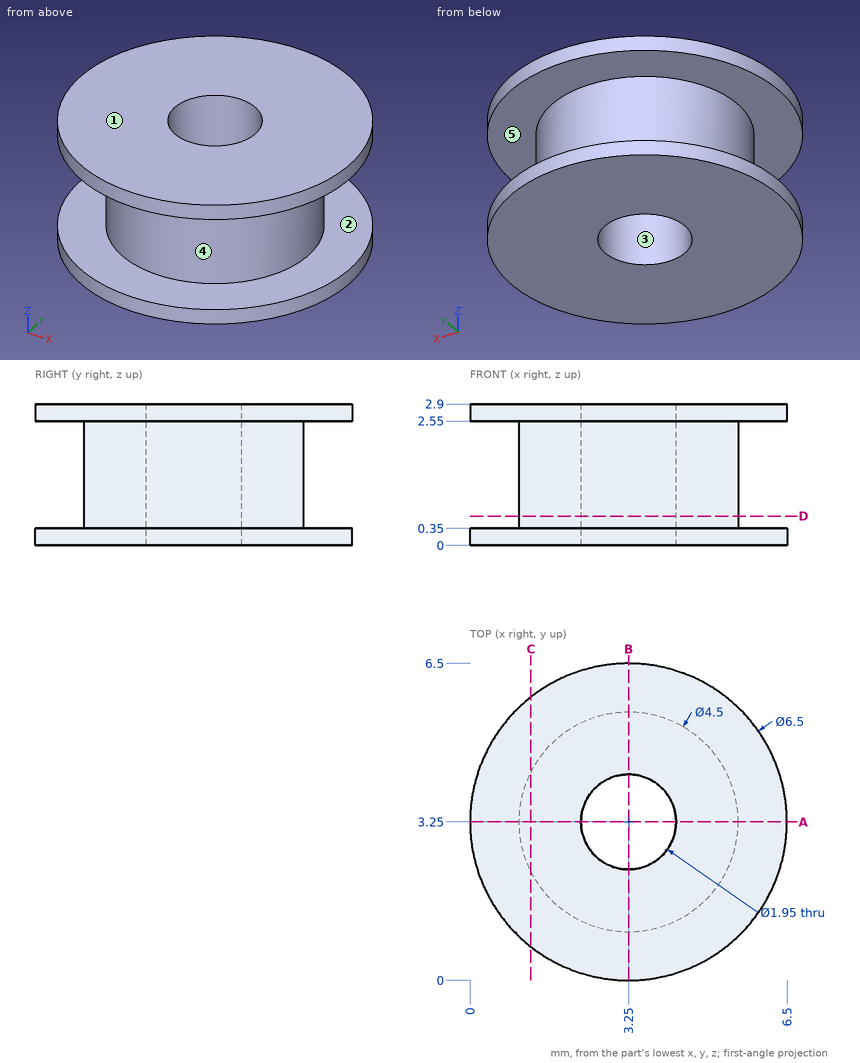
Design review of the part shown in the three views and the two pictorial views. Dimensions are in mm from the part's minimum x, y and z. A direction names the side the tool comes from. Give positions to 0.01 mm unless a question says otherwise; leave off trailing zeros. Loops run counter-clockwise (first coordinate to the right, second up) from the corner with the lowest first, then second, coordinate; pieces in that order, holes last. Notation, with made-up numbers: (64.5, 44.5) -> (77.5, 44.5) arc R19 ccw to (77.5, 71.5) -> close; hole circle Ø7 at (5, -36). An arc over 180 degrees is marked (long way). Write each question's results on one line, items separated by ' | '.
Q1. Take a section at D-D, the plane z = 0.6. Write out the cut boundary in (x, y) (3 decimals).
Reply:
outline: circle Ø4.5 at (3.25, 3.25); hole circle Ø1.95 at (3.25, 3.25)
Q2. Wall thickness on L1, parallel to Z at x = 5.5, y = 2.75; L2, parallel to Y at x = 3.25, z = 1.2 (3 decimals); L3, parallel to X at y = 3.75, z = 2.05: over which ranges is each line inside the solid? List them lowest first.
Reply:
L1: z = 0 to 0.35, 2.55 to 2.9 | L2: y = 1 to 2.275, 4.225 to 5.5 | L3: x = 1.06 to 2.41, 4.09 to 5.44
Q3. Machinability: for the marked faces 1 and 2, which of the approach directions +Z, -Z, +X, -X, +Y, -Y give a long, thin tool a straight path to every point of the face, cutting with its end or side? Answer none if there is none.
Reply:
face 1: +Z, +X, -X, +Y, -Y | face 2: none
Q4. The part is to be moulded in two halves that separate along X. For the marked faces 3, 4 and 5, say which applies: +X half, -X half, draft (parallel to the pull), parting line (faces both ways), or undercut.
Reply:
face 3: undercut | face 4: parting line | face 5: draft
Q5. Take a section at A-A, the plane y = 3.25. Write out the cut boundary in (x, z) (3 decimals).
Reply:
outline: (0, 0) -> (2.275, 0) -> (2.275, 2.9) -> (0, 2.9) -> (0, 2.55) -> (1, 2.55) -> (1, 0.35) -> (0, 0.35) -> close; (4.225, 0) -> (6.5, 0) -> (6.5, 0.35) -> (5.5, 0.35) -> (5.5, 2.55) -> (6.5, 2.55) -> (6.5, 2.9) -> (4.225, 2.9) -> close
Q6. For pin 1 Ø1.6 at (x, y) = (3.25, 3.25) entering from -Z, flat-tipped, find the tip position at first contact; note if it passes through.
Reply:
pin 1: passes through
Q7. Take a section at C-C, the plane x = 1.25. Write out the cut boundary in (y, z).
Reply:
outline: (0.69, 0) -> (5.81, 0) -> (5.81, 0.35) -> (4.28, 0.35) -> (4.28, 2.55) -> (5.81, 2.55) -> (5.81, 2.9) -> (0.69, 2.9) -> (0.69, 2.55) -> (2.22, 2.55) -> (2.22, 0.35) -> (0.69, 0.35) -> close
